Autodesk Inventor part; units mm, degrees
ref_plane "YZ Plane" through (0, 0, 0) normal (1, 0, 0) x (0, 1, 0)
ref_plane "XZ Plane" through (0, 0, 0) normal (0, 1, 0) x (-1, 0, 0)
ref_plane "XY Plane" through (0, 0, 0) normal (0, 0, 1) x (1, 0, 0)
sketch "Szkic1" plane through (0, 0, 0) normal (0, 0, 1) x (1, 0, 0)
  circle A0 centre (0, 0) radius 5.4
  line L0 (0, 5.4) -> (0, -12.6) construction
  line L1 (-5.4, 0) -> (-5.4, -12.6)
  line L2 (1.75, -12.6) -> (5.4, -12.6) construction
  line L3 (5.4, -12.6) -> (5.4, 0)
  line L4 (-4.5, -12.6) -> (-4.5, -16.6)
  line L5 (-4.5, -16.6) -> (-3, -16.6)
  line L6 (-3, -16.6) -> (-3, -13.6)
  line L7 (-3, -12.6) -> (-4.5, -12.6)
  line L8 (-4.5, -12.6) -> (-3, -16.6) construction
  line L9 (-4.5, -16.6) -> (-3, -12.6) construction
  line L10 (0.75, -12.6) -> (-0.75, -12.6)
  line L11 (0.75, -16.6) -> (0.75, -13.6)
  line L12 (-0.75, -16.6) -> (0.75, -16.6)
  line L13 (-0.75, -12.6) -> (0.75, -16.6) construction
  line L14 (-0.75, -16.6) -> (0.75, -12.6) construction
  line L15 (-0.75, -13.6) -> (-0.75, -16.6)
  line L16 (4.5, -12.6) -> (3, -12.6)
  line L17 (4.5, -16.6) -> (4.5, -12.6)
  line L18 (3, -16.6) -> (4.5, -16.6)
  line L19 (3, -12.6) -> (4.5, -16.6) construction
  line L20 (3, -16.6) -> (4.5, -12.6) construction
  line L21 (3, -13.6) -> (3, -16.6)
  line L22 (-7.5, 7.5) -> (7.5, 7.5)
  line L23 (7.5, 7.5) -> (7.5, -20.6)
  line L24 (7.5, -20.6) -> (-7.5, -20.6)
  line L25 (-7.5, -20.6) -> (-7.5, 7.5)
  line L26 (5.4, 0) -> (5.4, -20.6)
  line L27 (5.4, -20.6) -> (-5.4, -20.6) construction
  line L28 (-5.4, -20.6) -> (-5.4, 0)
  line L29 (-3, -16.6) -> (-3, -20.6)
  line L30 (-0.75, -16.6) -> (-0.75, -20.6)
  line L31 (0.75, -16.6) -> (0.75, -20.6)
  line L32 (3, -16.6) -> (3, -20.6)
  line L33 (4.5, -16.6) -> (4.5, -20.6) construction
  line L34 (2, -12.6) -> (0.75, -12.6) construction
  line L35 (-3, -12.6) -> (-1.75, -12.6) construction
  arc A1 (-2, -12.6) -> (-3, -13.6) centre (-2, -13.6) ccw
  arc A2 (-0.75, -13.6) -> (-1.75, -12.6) centre (-1.75, -13.6) ccw
  arc A3 (1.75, -12.6) -> (0.75, -13.6) centre (1.75, -13.6) ccw
  arc A4 (3, -13.6) -> (2, -12.6) centre (2, -13.6) ccw
  line L36 (-2, -12.6) -> (-1.75, -12.6)
  line L37 (1.75, -12.6) -> (2, -12.6)
  line L38 (3, -13.6) -> (3, -16.6)
  line L39 (5.4, -16.6) -> (3, -16.6) construction
  line L40 (-3, -16.6) -> (-5.4, -16.6) construction
  line L41 (-3, -16.6) -> (-3, -13.6)
  line L42 (-0.75, -13.6) -> (-0.75, -16.6)
  line L43 (0.75, -16.6) -> (0.75, -13.6)
  circle A5 centre (0, 0) radius 7.5
  line L44 (-7.5, -7.5) -> (7.5, -7.5)
  point P0 (-3.75, -14.6)
  point P1 (0, -14.6)
  point P2 (3.75, -14.6)
  point P3 (0, -14.6)
  point P4 (0, -14.6)
  point P5 (0, 5.4)
  point P6 (-3, -20.5)
  point P7 (-0.75, -20.6)
  point P8 (0.75, -13.6)
  point P9 (0.75, -20.6)
  point P10 (3, -20.6)
  point P11 (5.4, -12.6)
  point P12 (0, 7.5)
  point P13 (7.5, 0)
  point P14 (-7.5, 0)
  point P15 (-5.4, -5.2048)
  point P16 (5.4, -5.2048)
  dimension "d29" = 15
  dimension "d0" = 10.8
  dimension "d3" = 12.6
  dimension "d5" = 4
  dimension "d6" = 1.5
  dimension "d9" = 3.75
  dimension "d16" = 1
  dimension "d28" = 15
  dimension "d30" = 28.1
extrude "Wyciągnięcie proste1" add sketch "Szkic1" against normal blind 2 contours L3 A5 L1 A0 | A0 L1 A5 L3 | A5 L23 L44 L3 | L3 L44 A5 | A5 L44 L1 | L1 L44 L25 A5 | L44 L23 L24 L26 L3 | L3 L26 L24 L32 L21 A4 L37 A3 L11 L12 L15 A2 L36 A1 L6 L29 L28 L1 L44 | L1 L28 L24 L25 L44 | L24 L31 L11 A3 L37 A4 L21 L32 | L29 L6 A1 L36 A2 L15 L30 L24 | L24 L30 L12 L31
extrude "Wyciągnięcie proste2" add sketch "Szkic1" along normal blind 3 contours A0 L1 A5 L3 | A5 L23 L44 L3 | L1 L44 L25 A5 | L44 L23 L24 L26 L3 | L1 L28 L24 L25 L44 | L24 L31 L11 A3 L37 A4 L21 L32 | L29 L6 A1 L36 A2 L15 L30 L24 picked at (-5.6976, -3.095)
fillet "Zaokrąglenie1" radius 0.6 8 edges at (-7.5, -20.6, 0.5) (7.5, -20.6, 0.5) (-5.4, -20.6, 1.5) (5.4, -20.6, 1.5) (3, -20.6, 1.5) (0.75, -20.6, 1.5) (-3, -20.6, 1.5) (-0.75, -20.6, 1.5)
properties part number "potentiometr_case" material "PLA"
Here's how the part is built. I have some questions about the finished solid (model axes, mm). A direction names the side the tool comes from. Round coordinates to 2 decimals unless told otherwise and drop trailing zeros. Order: outer loops, then holes, each group sorted by start corner. A loop starts at its lowest first (then second) coordinate and runs counter-clockwise, first axis right, second up. Notation, with made-up numbers: (-1, -4) -> (21, -4) arc R20 ccw to (21, 25) -> close; hole circle Ø3 at (74.5, 60.25). An arc over 180 degrees is marked (long way). Use CSV: the item, a comma, the result in double quotes.
1. I want a section at A-A on x = 0. List the corners of the cut face in (y, z) for me.
Recorded:
outline,"(-20.6, -2) -> (-5.4, -2) -> (-5.4, 0) -> (-20.6, 0) -> close; (5.4, -2) -> (7.5, -2) -> (7.5, 3) -> (5.4, 3) -> close"
2. I want a section at B-B on z = -1. List the corners of the cut face in (x, y) for me.
Recorded:
outline,"(-7.5, -20) arc R0.6 ccw to (-6.9, -20.6) -> (6.9, -20.6) arc R0.6 ccw to (7.5, -20) -> (7.5, 0) arc R7.5 ccw to (-7.5, 0) -> close; hole circle Ø10.8 at (0, 0)"
3. Thinking about a two-plate mould opening in X: for faces 1 (the face through (0.75, -17, 1)), 2 (the face through (0, -9, -2)), 3 (the face through (-7.5, -10, 1)), 4 (the face through (0.16, 7.5, 0.54)), which applies, pulls with the +X half, pulls with the -X half, needs draft (parallel to the pull), parting line crosses it, or undercut?
Recorded:
face 1,"undercut"
face 2,"needs draft"
face 3,"pulls with the -X half"
face 4,"parting line crosses it"
4. I need wall thicknesses on line 1 along X through (y, z) = (-18.5, 2); line 2 along X through (y, z) = (-9.5, 2.15); line 3 along Y through (x, z) = (0, 0.5). Which ranges of each line are inside material? Lowest first, please.
Recorded:
line 1,"x = -7.5 to -5.4, -3 to -0.75, 0.75 to 3, 5.4 to 7.5"
line 2,"x = -7.5 to -5.4, 5.4 to 7.5"
line 3,"y = 5.4 to 7.5"
5. Which directions (+Z, -Z, +X, -X, +Y, -Y) give clear straight access to the entire face, cutting with the end or side of a thin tool? Please do faces 5 (the face through (-1.051, -12.885, 1.479)), 6 (the face through (-3, -17, 1)), 7 (the face through (7.5, -10, 1)).
Recorded:
face 5,"+Z"
face 6,"+Z, -Y"
face 7,"+Z, -Z, +X, +Y, -Y"
6. I want a section at D-D on y = -3. List the corners of the cut face in (x, z) for me.
Recorded:
outline,"(-7.5, -2) -> (-4.49, -2) -> (-4.49, 0) -> (-5.4, 0) -> (-5.4, 3) -> (-7.5, 3) -> close; (4.49, -2) -> (7.5, -2) -> (7.5, 3) -> (5.4, 3) -> (5.4, 0) -> (4.49, 0) -> close"
7. I want a section at C-C on z = 0.3. List the corners of the cut face in (x, y) for me, and give its area (3 significant figures).
Recorded:
outline,"(-7.5, -20) arc R0.6 ccw to (-6.9, -20.6) -> (-6, -20.6) arc R0.6 ccw to (-5.4, -20) -> (-5.4, 0) arc R5.4 cw to (5.4, 0) -> (5.4, -20) arc R0.6 ccw to (6, -20.6) -> (6.9, -20.6) arc R0.6 ccw to (7.5, -20) -> (7.5, 0) arc R7.5 ccw to (-7.5, 0) -> close; (-3, -20) arc R0.6 ccw to (-2.4, -20.6) -> (-1.35, -20.6) arc R0.6 ccw to (-0.75, -20) -> (-0.75, -13.6) arc R1 ccw to (-1.75, -12.6) -> (-2, -12.6) arc R1 ccw to (-3, -13.6) -> close; (0.75, -20) arc R0.6 ccw to (1.35, -20.6) -> (2.4, -20.6) arc R0.6 ccw to (3, -20) -> (3, -13.6) arc R1 ccw to (2, -12.6) -> (1.75, -12.6) arc R1 ccw to (0.75, -13.6) -> close"
area,"164 mm2"
